```python
from build123d import *

# Parameters (mm, degrees)
F0_W     = 215.9
F0_H     = 273.05
F0_W_2   = 50.8
F0_H_2   = 19.05
F1_DEPTH = 6.35


with BuildPart() as f1:
    # F0 (on Front) → F1 (new body)
    with BuildSketch(Plane.XZ):
        with Locations((0, 136.525)):
            Rectangle(F0_W, F0_H)
        with Locations((-63.5, 47.625)):
            Rectangle(F0_W_2, F0_H_2, mode=Mode.SUBTRACT)
        with Locations((-63.5, 79.375)):
            Rectangle(F0_W_2, F0_H_2, mode=Mode.SUBTRACT)
        with Locations((-63.5, 111.125)):
            Rectangle(F0_W_2, F0_H_2, mode=Mode.SUBTRACT)
        with Locations((0, 47.625)):
            Rectangle(F0_W_2, F0_H_2, mode=Mode.SUBTRACT)
        with Locations((63.5, 47.625)):
            Rectangle(F0_W_2, F0_H_2, mode=Mode.SUBTRACT)
        with Locations((0, 79.375)):
            Rectangle(F0_W_2, F0_H_2, mode=Mode.SUBTRACT)
        with Locations((0, 111.125)):
            Rectangle(F0_W_2, F0_H_2, mode=Mode.SUBTRACT)
        with Locations((63.5, 79.375)):
            Rectangle(F0_W_2, F0_H_2, mode=Mode.SUBTRACT)
        with Locations((63.5, 111.125)):
            Rectangle(F0_W_2, F0_H_2, mode=Mode.SUBTRACT)
        with Locations((-63.5, 142.875)):
            Rectangle(F0_W_2, F0_H_2, mode=Mode.SUBTRACT)
        with Locations((-63.5, 174.625)):
            Rectangle(F0_W_2, F0_H_2, mode=Mode.SUBTRACT)
        with Locations((0, 142.875)):
            Rectangle(F0_W_2, F0_H_2, mode=Mode.SUBTRACT)
        with Locations((0, 174.625)):
            Rectangle(F0_W_2, F0_H_2, mode=Mode.SUBTRACT)
        with Locations((63.5, 142.875)):
            Rectangle(F0_W_2, F0_H_2, mode=Mode.SUBTRACT)
        with Locations((63.5, 174.625)):
            Rectangle(F0_W_2, F0_H_2, mode=Mode.SUBTRACT)
    extrude(amount=F1_DEPTH)


solid = f1.part
```
Source: CAD feature listing. Evaluate the final solid. Frame: model axes, mm. Round coordinates to 2 decimals unless told otherwise and drop trailing zeros. Write each loop counter-clockwise with the first axis right and the second up, starting at its lowest first coordinate (ties: lowest second). Pieces come first, ordered by that corner, then holes. Notation, with made-up numbers: M -22.75,60.25 L 9.25,60.25 A16 ccw 9.25,67.25 Z; hole C -32,5.5 d11. An arc over 180 degrees is marked long. Use CSV: the item, a comma, the result in double quotes. Start each with the question number.
Q1. Cut plane A-A on z = 107. Output: boundary loops of the cut face in (x, y).
Q2. Pull-direction query (X, two-part tool) for faces 1 (the face through (-88.9, -3, 79)), 2 (the face through (-2, -3, 0)); classes: +X half, -X half, draft (parallel to the pull), parting line (faces both ways), or undercut.
Q3. First-contact query: P1, Ø6, axis at x = 67, z = 88, coming from the +Y side. Flat tip, straight axial feed; report the tip coordinate or a pass-through.
Q4. Cut plane C-C on y = -5. Count the separate pieces of the cut face and the enclosed holes in it, plus the area to 3 significant figures.
Q5. Line query: line 1 (Z direction, x = 45.5, y = -0.5); line 2 (X direction, y = -1.5, z = 80.5). Output: solid intervals per line, ascending. Write a range as from..to.
Q6. Cut plane B-B on x = 19. Output: boundary loops of the cut face in (y, z), plus the area to 3 significant figures.
Results found:
1,outline,"M -107.95,-6.35 L -88.9,-6.35 L -88.9,0 L -107.95,0 Z; M -38.1,-6.35 L -25.4,-6.35 L -25.4,0 L -38.1,0 Z; M 25.4,-6.35 L 38.1,-6.35 L 38.1,0 L 25.4,0 Z; M 88.9,-6.35 L 107.95,-6.35 L 107.95,0 L 88.9,0 Z"
2,face 1,"undercut"
2,face 2,"draft"
3,P1,"y = 0"
4,separate pieces,"1"
4,enclosed holes,"15"
4,area,"44,400 mm^2"
5,line 1,"0..38.1, 57.15..69.85, 88.9..101.6, 120.65..133.35, 152.4..165.1, 184.15..273.05"
5,line 2,"-107.95..-88.9, -38.1..-25.4, 25.4..38.1, 88.9..107.95"
6,outline,"M -6.35,0 L 0,0 L 0,38.1 L -6.35,38.1 Z; M -6.35,57.15 L 0,57.15 L 0,69.85 L -6.35,69.85 Z; M -6.35,88.9 L 0,88.9 L 0,101.6 L -6.35,101.6 Z; M -6.35,120.65 L 0,120.65 L 0,133.35 L -6.35,133.35 Z; M -6.35,152.4 L 0,152.4 L 0,165.1 L -6.35,165.1 Z; M -6.35,184.15 L 0,184.15 L 0,273.05 L -6.35,273.05 Z"
6,area,"1,130 mm^2"
